The drawing under review shows one solid part. Ordinate dimensions are in mm from its lowest x, y, z. A direction names the side the tool comes from. Give positions to 0.01 mm unless a question says otherwise; leave off trailing zeros. Write each loop counter-clockwise with the first axis right and the second up, starting at its lowest first coordinate (ties: lowest second). Pieces come first, ordered by that corner, then holes. Notation, with made-up numbers: (35, -7) -> (40, -7) arc R35 cw to (40, 32) -> close; hole circle Ø1 at (29, -19). An arc over 180 degrees is marked (long way). Write item = value, one per line.
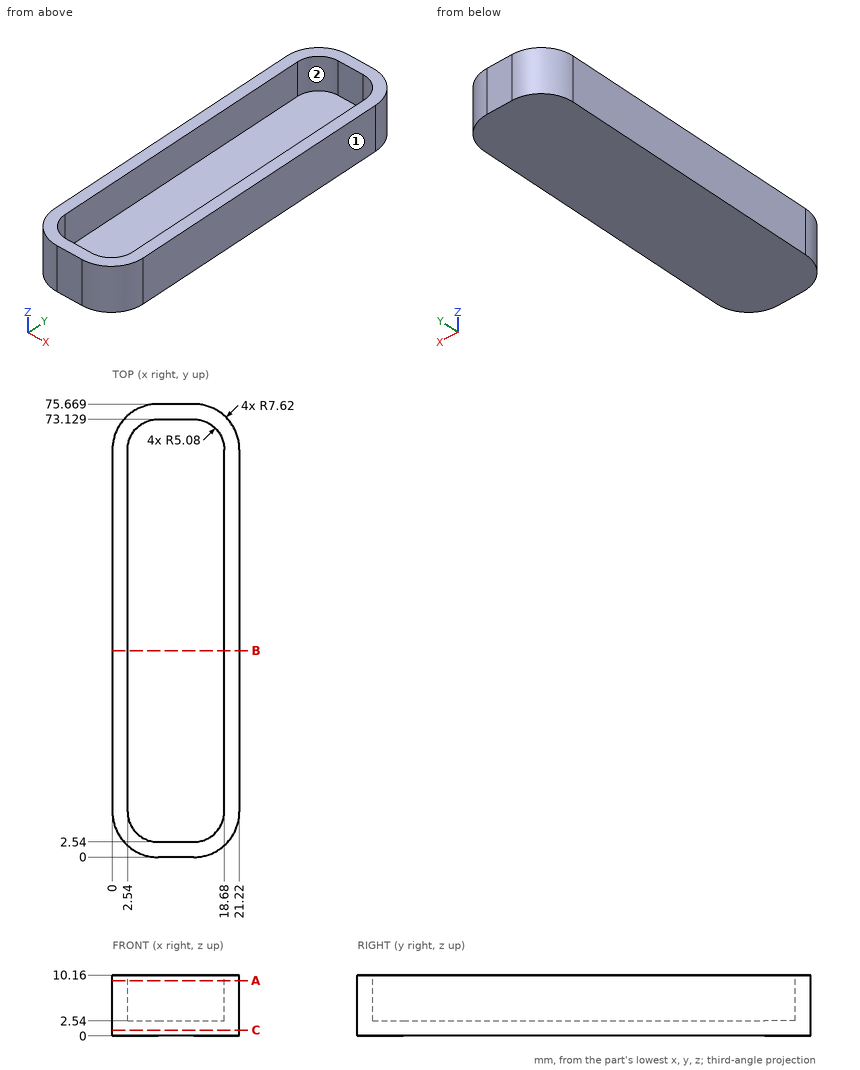
(1) To check wall thickness, follow probe 1 along X at (y, z) = (39, 7); probe 2 along Y at (x, z) = (9.5, 7); probe 3 along Z at (x, y) = (7.25, 56.5). State the ranges of each line that lie inside material, in increasing order.
Answers below:
probe_1 = 0 to 2.54, 18.68 to 21.22
probe_2 = 0 to 2.54, 73.13 to 75.67
probe_3 = 0 to 2.54
(2) For pin 1 (8 mm diameter, centred on x = 7.5, y = 38, fed in from +Z); pin 2 (4 mm diameter, centred on x = 6, y = 19.5, fed in from -Z), all flat-tipped, find the tip position at first contact; note any pin that passes through.
Answers below:
pin_1 = 2.54
pin_2 = 0
(3) Take a section at A-A (z = 9.25). Write out the cut boundary in (x, y).
Answers below:
outline = (0, 7.62) arc R7.62 ccw to (7.62, 0) -> (13.6, 0) arc R7.62 ccw to (21.22, 7.62) -> (21.22, 68.05) arc R7.62 ccw to (13.6, 75.67) -> (7.62, 75.67) arc R7.62 ccw to (0, 68.05) -> close; hole (2.54, 7.62) arc R5.08 ccw to (7.62, 2.54) -> (13.6, 2.54) arc R5.08 ccw to (18.68, 7.62) -> (18.68, 68.05) arc R5.08 ccw to (13.6, 73.13) -> (7.62, 73.13) arc R5.08 ccw to (2.54, 68.05) -> close
(4) Take a section at B-B (y = 34.5). Write out the cut boundary in (x, z).
Answers below:
outline = (0, 0) -> (21.22, 0) -> (21.22, 10.16) -> (18.68, 10.16) -> (18.68, 2.54) -> (2.54, 2.54) -> (2.54, 10.16) -> (0, 10.16) -> close
(5) Tool access review of the marked faces 1 and 2: name each direction out of +Z, -Z, +X, -X, +Y, -Y from which nothing blocks a thin tool from reaching the whole face with its end or side.
Answers below:
face_1 = +Z, -Z, +X, +Y, -Y
face_2 = +Z
(6) Take a section at C-C (z = 1). Write out the cut boundary in (x, y), plus the area to 3 significant figures.
Answers below:
outline = (0, 7.62) arc R7.62 ccw to (7.62, 0) -> (13.6, 0) arc R7.62 ccw to (21.22, 7.62) -> (21.22, 68.05) arc R7.62 ccw to (13.6, 75.67) -> (7.62, 75.67) arc R7.62 ccw to (0, 68.05) -> close
area = 1,560 mm^2
